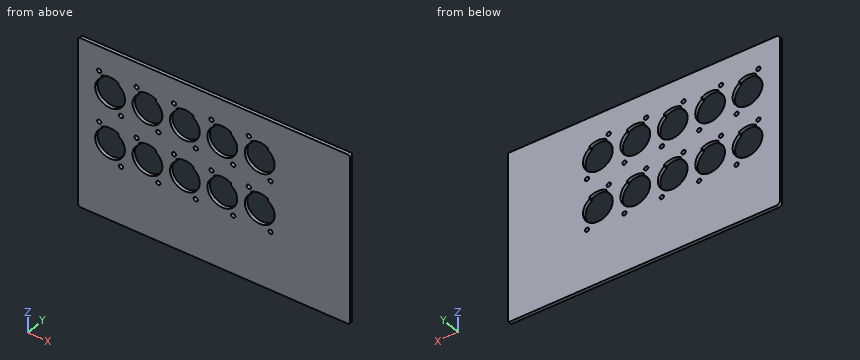
from build123d import *

# Parameters (mm, degrees)
F0_R     = 1.5875
F1_DEPTH = 2.54


with BuildPart() as f1:
    # F0 (on Front) → F1 (new body)
    with BuildSketch(Plane.XZ):
        with BuildLine():
            Line((93.98, 52.134603), (-105.41, 52.134603))
            ThreePointArc((-105.41, 52.134603), (-107.206051, 51.390655), (-107.95, 49.594603))
            Line((-107.95, 49.594603), (-107.95, -75.500397))
            ThreePointArc((-107.95, -75.500397), (-107.206051, -77.296448), (-105.41, -78.040397))
            Line((-105.41, -78.040397), (93.98, -78.040397))
            ThreePointArc((93.98, -78.040397), (94.878026, -77.668422), (95.25, -76.770397))
            Line((95.25, -76.770397), (95.25, 50.864603))
            ThreePointArc((95.25, 50.864603), (94.878026, 51.762629), (93.98, 52.134603))
        make_face()
        with Locations((-75.692, -33.2105)):
            Circle(F0_R, mode=Mode.SUBTRACT)
        with BuildLine():
            ThreePointArc((-77.47, -10.406757), (-83.82, -30.63875), (-90.17, -10.406757))
            Line((-90.17, -10.406757), (-90.17, -8.817245))
            ThreePointArc((-90.17, -8.817245), (-83.82, -7.076138), (-77.47, -8.817245))
            Line((-77.47, -8.817245), (-77.47, -10.406757))
        make_face(mode=Mode.SUBTRACT)
        with Locations((-47.752, -33.2105)):
            Circle(F0_R, mode=Mode.SUBTRACT)
        with Locations((-19.812, -33.2105)):
            Circle(F0_R, mode=Mode.SUBTRACT)
        with BuildLine():
            ThreePointArc((-49.53, -10.406757), (-55.88, -30.63875), (-62.23, -10.406757))
            Line((-62.23, -10.406757), (-62.23, -8.817245))
            ThreePointArc((-62.23, -8.817245), (-55.88, -7.076138), (-49.53, -8.817245))
            Line((-49.53, -8.817245), (-49.53, -10.406757))
        make_face(mode=Mode.SUBTRACT)
        with BuildLine():
            ThreePointArc((-21.59, -10.406757), (-27.94, -30.63875), (-34.29, -10.406757))
            Line((-34.29, -10.406757), (-34.29, -8.817245))
            ThreePointArc((-34.29, -8.817245), (-27.94, -7.076138), (-21.59, -8.817245))
            Line((-21.59, -8.817245), (-21.59, -10.406757))
        make_face(mode=Mode.SUBTRACT)
        with Locations((8.128, -33.2105)):
            Circle(F0_R, mode=Mode.SUBTRACT)
        with Locations((36.068, -33.2105)):
            Circle(F0_R, mode=Mode.SUBTRACT)
        with BuildLine():
            ThreePointArc((6.35, -10.406757), (0, -30.63875), (-6.35, -10.406757))
            Line((-6.35, -10.406757), (-6.35, -8.817245))
            ThreePointArc((-6.35, -8.817245), (0, -7.076138), (6.35, -8.817245))
            Line((6.35, -8.817245), (6.35, -10.406757))
        make_face(mode=Mode.SUBTRACT)
        with BuildLine():
            ThreePointArc((34.29, -10.406757), (27.94, -30.63875), (21.59, -10.406757))
            Line((21.59, -10.406757), (21.59, -8.817245))
            ThreePointArc((21.59, -8.817245), (27.94, -7.076138), (34.29, -8.817245))
            Line((34.29, -8.817245), (34.29, -10.406757))
        make_face(mode=Mode.SUBTRACT)
        with Locations((-91.948, -5.842)):
            Circle(F0_R, mode=Mode.SUBTRACT)
        with Locations((-64.008, -5.842)):
            Circle(F0_R, mode=Mode.SUBTRACT)
        with Locations((-75.692, 5.842)):
            Circle(F0_R, mode=Mode.SUBTRACT)
        with Locations((-36.068, -5.842)):
            Circle(F0_R, mode=Mode.SUBTRACT)
        with Locations((-8.128, -5.842)):
            Circle(F0_R, mode=Mode.SUBTRACT)
        with Locations((-47.752, 5.842)):
            Circle(F0_R, mode=Mode.SUBTRACT)
        with Locations((-19.812, 5.842)):
            Circle(F0_R, mode=Mode.SUBTRACT)
        with BuildLine():
            ThreePointArc((-77.47, 28.645743), (-83.82, 8.41375), (-90.17, 28.645743))
            Line((-90.17, 28.645743), (-90.17, 30.235255))
            ThreePointArc((-90.17, 30.235255), (-83.82, 31.976362), (-77.47, 30.235255))
            Line((-77.47, 30.235255), (-77.47, 28.645743))
        make_face(mode=Mode.SUBTRACT)
        with Locations((-91.948, 33.2105)):
            Circle(F0_R, mode=Mode.SUBTRACT)
        with Locations((-64.008, 33.2105)):
            Circle(F0_R, mode=Mode.SUBTRACT)
        with BuildLine():
            ThreePointArc((-49.53, 28.645743), (-55.88, 8.41375), (-62.23, 28.645743))
            Line((-62.23, 28.645743), (-62.23, 30.235255))
            ThreePointArc((-62.23, 30.235255), (-55.88, 31.976362), (-49.53, 30.235255))
            Line((-49.53, 30.235255), (-49.53, 28.645743))
        make_face(mode=Mode.SUBTRACT)
        with Locations((-36.068, 33.2105)):
            Circle(F0_R, mode=Mode.SUBTRACT)
        with BuildLine():
            ThreePointArc((-21.59, 28.645743), (-27.94, 8.41375), (-34.29, 28.645743))
            Line((-34.29, 28.645743), (-34.29, 30.235255))
            ThreePointArc((-34.29, 30.235255), (-27.94, 31.976362), (-21.59, 30.235255))
            Line((-21.59, 30.235255), (-21.59, 28.645743))
        make_face(mode=Mode.SUBTRACT)
        with Locations((-8.128, 33.2105)):
            Circle(F0_R, mode=Mode.SUBTRACT)
        with Locations((19.812, -5.842)):
            Circle(F0_R, mode=Mode.SUBTRACT)
        with Locations((8.128, 5.842)):
            Circle(F0_R, mode=Mode.SUBTRACT)
        with Locations((36.068, 5.842)):
            Circle(F0_R, mode=Mode.SUBTRACT)
        with BuildLine():
            ThreePointArc((6.35, 28.645743), (0, 8.41375), (-6.35, 28.645743))
            Line((-6.35, 28.645743), (-6.35, 30.235255))
            ThreePointArc((-6.35, 30.235255), (0, 31.976362), (6.35, 30.235255))
            Line((6.35, 30.235255), (6.35, 28.645743))
        make_face(mode=Mode.SUBTRACT)
        with BuildLine():
            ThreePointArc((34.29, 28.645743), (27.94, 8.41375), (21.59, 28.645743))
            Line((21.59, 28.645743), (21.59, 30.235255))
            ThreePointArc((21.59, 30.235255), (27.94, 31.976362), (34.29, 30.235255))
            Line((34.29, 30.235255), (34.29, 28.645743))
        make_face(mode=Mode.SUBTRACT)
        with Locations((19.812, 33.2105)):
            Circle(F0_R, mode=Mode.SUBTRACT)
    extrude(amount=F1_DEPTH)


solid = f1.part
Can you work these out from the model? Positions are in its coordinate system, mm. Coordinates: 2 decimals unless noted, no trailing zeros. Loops run counter-clockwise (first coordinate to the right, second up) from the corner with the lowest first, then second, coordinate; pieces in that order, holes last. Notation, with made-up numbers: (67.25, 77) - (72.25, 77) arc R14 cw to (72.25, 101) - close; hole circle Ø4 at (85, -36). An arc over 180 degrees is marked (long way). Put each result on its own line as item: value. Start each with the question number.
Item 1: Suppose I cut it at B-B (x = -1). Please give me the cut outline in (y, z), and give its area (3 significant figures).
Item 2: Suppose I cut it at A-A (x = -27.94). Please give me the cut outline in (y, z).
Item 3: If I drill on line 1 along X through (y, z) = (-0.65, 25); line 2 along X through (y, z) = (-1.8, 33); line 3 along Z through (x, y) = (-56.5, -0.05), over which ranges is the centre line in solid material (lowest first)?
Item 4: Suppose I cut it at C-C (y = -1.45). State how many separate pieces and enclosed holes the cut face has, and give its area (3 significant figures).
Item 5: For pin 1 (1.9 mm diameter, centred on x = -64.008, z = -5.842, fed in from -Y), with a flat end and sliding along its axis, tell me the tip position at first contact or that it passes through.
Here are the results:
1. outline: (-2.54, -78.04) - (0, -78.04) - (0, -30.59) - (-2.54, -30.59) - close; (-2.54, -7.12) - (0, -7.12) - (0, 8.46) - (-2.54, 8.46) - close; (-2.54, 31.94) - (0, 31.94) - (0, 52.13) - (-2.54, 52.13) - close
1. area: 211 mm²
2. outline: (-2.54, -78.04) - (0, -78.04) - (0, -30.64) - (-2.54, -30.64) - close; (-2.54, -7.08) - (0, -7.08) - (0, 8.41) - (-2.54, 8.41) - close; (-2.54, 31.98) - (0, 31.98) - (0, 52.13) - (-2.54, 52.13) - close
3. line 1: -107.95 to -93.49, -74.15 to -65.55, -46.21 to -37.61, -18.27 to -9.67, 9.67 to 18.27, 37.61 to 95.25
3. line 2: -107.95 to -93.52, -90.37 to -65.58, -62.43 to -37.64, -34.49 to -9.7, -6.55 to 18.24, 21.39 to 95.25
3. line 3: -78.04 to -30.62, -7.09 to 8.43, 31.96 to 52.13
4. separate pieces: 1
4. enclosed holes: 30
4. area: 22,200 mm²
5. pin 1: through
